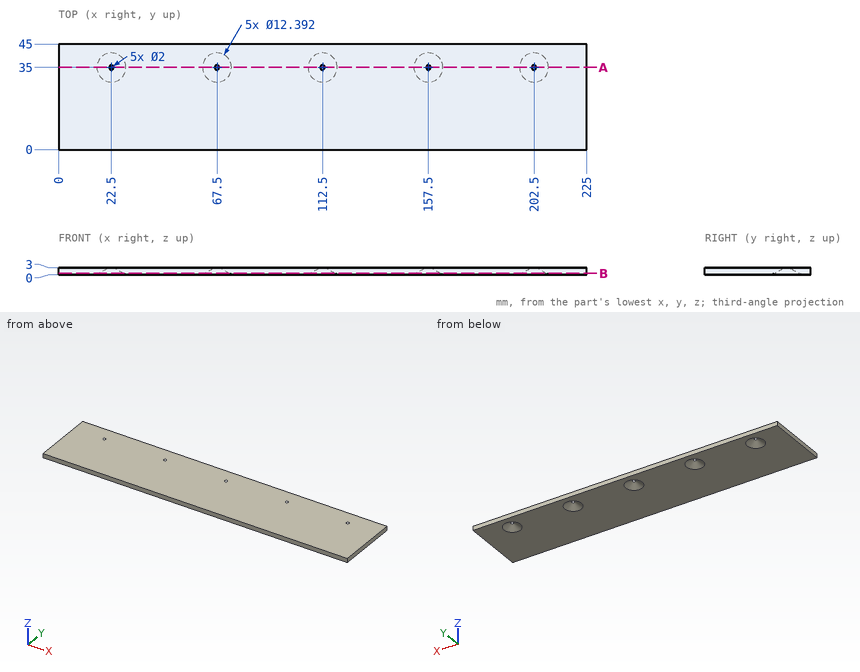
The drawing under review shows one solid part. Ordinate dimensions are in mm from its lowest x, y, z. Coordinates: 2 decimals unless noted, no trailing zeros. Write each loop counter-clockwise with the first axis right and the second up, starting at its lowest first coordinate (ties: lowest second). Pieces come first, ordered by that corner, then holes.
1) Add section A-A (y = 35). Write out the cut boundary in (x, z), plus the area to 3 significant figures.
2) Add section B-B (z = 0.55). Write out the cut boundary in (x, y), plus the area to 3 significant figures.
3) To check wall thickness, follow L1, parallel to X at y = 34, z = 1.9 (1 decimal); L2, parallel to Y at x = 22.5, z = 0.8; L3, parallel to Y at x = 22.5, z = 2.6 (1 decimal). State the ranges of each line that lie inside material, in increasing order.
Check result:
1. outline: (0, 0) - (16.3, 0) - (21.5, 3) - (0, 3) - close; (23.5, 3) - (28.7, 0) - (61.3, 0) - (66.5, 3) - close; (68.5, 3) - (73.7, 0) - (106.3, 0) - (111.5, 3) - close; (113.5, 3) - (118.7, 0) - (151.3, 0) - (156.5, 3) - close; (158.5, 3) - (163.7, 0) - (196.3, 0) - (201.5, 3) - close; (203.5, 3) - (208.7, 0) - (225, 0) - (225, 3) - close
1. area: 567 mm2
2. outline: (0, 0) - (225, 0) - (225, 45) - (0, 45) - close; hole circle Ø10.49 at (22.5, 35); hole circle Ø10.49 at (67.5, 35); hole circle Ø10.49 at (112.5, 35); hole circle Ø10.49 at (157.5, 35); hole circle Ø10.49 at (202.5, 35)
2. area: 9,690 mm2
3. L1: x = 0 to 19.8, 25.2 to 64.8, 70.2 to 109.8, 115.2 to 154.8, 160.2 to 199.8, 205.2 to 225
3. L2: y = 0 to 30.19, 39.81 to 45
3. L3: y = 0 to 33.3, 36.7 to 45
